Source: CAD feature listing. Evaluate the final solid. Frame: model axes, mm. Round coordinates to 2 decimals unless told otherwise and drop trailing zeros. Write each loop counter-clockwise with the first axis right and the second up, starting at its lowest first coordinate (ties: lowest second). Pieces come first, ordered by that corner, then holes.
```python
from build123d import *

# Parameters (mm, degrees)
SKETCH1_W           = 310.792155558
SKETCH1_H           = 307.10414309
BOSS_EXTRUDE1_DEPTH = 3.175
SKETCH2_W           = 302.308555558
SKETCH2_H           = 298.62054309
BOSS_EXTRUDE2_DEPTH = 1.27
BOSS_EXTRUDE4_DEPTH = 3.175
SKETCH6_R           = 0.911045746
SKETCH6_R_2         = 1.683740392
BOSS_EXTRUDE7_DEPTH = 0.254
SKETCH7_R           = 3.556
BOSS_EXTRUDE8_DEPTH = 23.876


with BuildPart() as part:
    # Sketch1 → Boss-Extrude1 (new body)
    with BuildSketch(Plane(origin=(0, 0, 0), x_dir=(1, 0, 0), z_dir=(0, 1, 0))):
        Rectangle(SKETCH1_W, SKETCH1_H)
    extrude(amount=BOSS_EXTRUDE1_DEPTH)

    # Sketch2 → Boss-Extrude2 (add)
    with BuildSketch(Plane(origin=(0, 3.175, 0), x_dir=(1, 0, 0), z_dir=(0, 1, 0))):
        Rectangle(SKETCH2_W, SKETCH2_H)
    extrude(amount=BOSS_EXTRUDE2_DEPTH)



with BuildPart() as body_2:
    # 3DSketch1 → Boss-Extrude4 (new body)
    with BuildSketch(Plane(origin=(-155.396077779, 25.1714, -153.552071545), x_dir=(0.7113145904869971, 0, 0.7028737819554204), z_dir=(0, -1, 0))):
        Polygon((0, 0), (215.855450508, 218.447657779), (436.926445365, 0), (221.070994857, -218.447657779), align=None)
    extrude(amount=BOSS_EXTRUDE4_DEPTH)

    # Sketch6 → Boss-Extrude7 (add)
    with BuildSketch(Plane(origin=(0, 25.1714, 0), x_dir=(1, 0, 0), z_dir=(0, 1, 0))):
        with Locations(Location((-60.146077779, -108.71629912, 0), (0, 0, 90))):
            Circle(SKETCH6_R)
        with Locations(Location((-21.538077779, -66.55229912, 0), (0, 0, 90))):
            Circle(SKETCH6_R_2)
        with Locations(Location((-60.146077779, 108.71629912, 0), (0, 0, 90))):
            Circle(SKETCH6_R)
        with Locations(Location((-21.538077779, 66.55229912, 0), (0, 0, 90))):
            Circle(SKETCH6_R_2)
        with Locations(Location((21.538077779, 66.55229912, 0), (0, 0, 90))):
            Circle(SKETCH6_R_2)
        with Locations(Location((60.146077779, 108.71629912, 0), (0, 0, 90))):
            Circle(SKETCH6_R)
        with Locations(Location((21.538077779, -66.55229912, 0), (0, 0, 90))):
            Circle(SKETCH6_R_2)
        with Locations(Location((60.146077779, -108.71629912, 0), (0, 0, 90))):
            Circle(SKETCH6_R)
    extrude(amount=BOSS_EXTRUDE7_DEPTH)


with BuildPart() as part_1:
    add(part.part)

    add(body_2.part)  # Boss-Extrude8 merges body 2
    # Sketch7 → Boss-Extrude8 (add)
    with BuildSketch(Plane.XZ):
        with Locations(Location((-150.316077779, 148.472071545, 0), (0, 0, 270))):
            Circle(SKETCH7_R)
        with Locations(Location((150.316077779, 148.472071545, 0), (0, 0, 270))):
            Circle(SKETCH7_R)
        with Locations(Location((150.316077779, -148.472071545, 0), (0, 0, 270))):
            Circle(SKETCH7_R)
        with Locations(Location((-150.316077779, -148.472071545, 0), (0, 0, 270))):
            Circle(SKETCH7_R)
    extrude(amount=-BOSS_EXTRUDE8_DEPTH)


solid = part_1.part
```
Q1. Mould query, pull axis Y, two halves, no side actions, for faces 1 (the face through (0, 25.171, 4)), 2 (the face through (0, 21.996, 4)), 3 (the face through (2, 0, 2)). Classes: pulls with the +Y half, pulls with the -Y half, needs draft (parallel to the pull), parting line crosses it, or undercut.
Q2. Section query A-A, the plane x = -1. Output: boundary loops of the cut face in (y, z) (3 decimals).
Q3. Line query: line 1 (Y direction, x = 96.5, z = -113.5) (3 decimals). Output: solid intervals per line, ascending.
Q4. Pin query (flat end, axial travel): P1, Ø0.6, axis at y = 4, z = 44, coming from the +X side; P2, Ø1.4, axis at x = 28.5, y = 4, coming from the -Z side; P3, Ø5, axis at x = -66, z = 73.5, coming from the +Y side. Return the tip coordinate at first contact, or that it passes through.
Q5. Section query B-B, the plane z = 119. Output: boundary loops of the cut face in (x, y) (3 decimals).
Q6. Section query C-C, the plane y = 14.25. Output: boundary loops of the cut face in (x, z).
Filled in:
1. face 1: pulls with the +Y half
1. face 2: undercut
1. face 3: pulls with the -Y half
2. outline: (0, -153.552) - (3.175, -153.552) - (3.175, -149.31) - (4.445, -149.31) - (4.445, 149.31) - (3.175, 149.31) - (3.175, 153.552) - (0, 153.552) - close; (21.996, -153.552) - (25.171, -153.552) - (25.171, 153.552) - (21.996, 153.552) - close
3. line 1: y = 0 to 4.445, 21.996 to 25.171
4. P1: stops at x = 151.15
4. P2: stops at z = -149.31
4. P3: stops at y = 25.17
5. outline: (-155.396, 0) - (155.396, 0) - (155.396, 3.175) - (151.154, 3.175) - (151.154, 4.445) - (-151.154, 4.445) - (-151.154, 3.175) - (-155.396, 3.175) - close; (-155.396, 21.996) - (155.396, 21.996) - (155.396, 25.171) - (-155.396, 25.171) - close
6. outline: circle Ø7.11 at (-150.32, -148.47); circle Ø7.11 at (-150.32, 148.47); circle Ø7.11 at (150.32, -148.47); circle Ø7.11 at (150.32, 148.47)
